Source: CAD feature listing. Evaluate the final solid. Frame: model axes, mm. A direction names the side the tool comes from. Coordinates: 2 decimals unless noted, no trailing zeros. Loops run counter-clockwise (first coordinate to the right, second up) from the corner with the lowest first, then second, coordinate; pieces in that order, holes last. Notation, with made-up numbers: (-2, -7) -> (4, -7) arc R10 cw to (4, 4) -> close; hole circle Ø6 at (67, 42.25). An arc over 180 degrees is marked (long way). Answer as a JSON object with one key per item and string values. Group by question number.
from build123d import *


with BuildPart() as part:
    # Sketch1 → Revolve1 (revolve)
    with BuildSketch(Plane.XY, mode=Mode.PRIVATE) as revolve1_sk:
        with BuildLine():
            Line((0, 76.2), (-7.9375, 76.2))
            Line((-7.9375, 76.2), (-7.9375, 64.29375))
            ThreePointArc((-7.9375, 64.29375), (-8.169983992, 63.732483992), (-8.73125, 63.5))
            Line((-8.73125, 63.5), (-12.7, 63.5))
            Line((-12.7, 63.5), (-12.7, -63.5))
            Line((-12.7, -63.5), (-8.73125, -63.5))
            ThreePointArc((-8.73125, -63.5), (-8.169983992, -63.732483992), (-7.9375, -64.29375))
            Line((-7.9375, -64.29375), (-7.9375, -76.2))
            Line((-7.9375, -76.2), (0, -76.2))
            Line((0, -76.2), (0, 76.2))
        make_face()
    revolve(revolve1_sk.sketch.rotate(Axis((0, 76.2, 0), (0, -1, 0)), 270), axis=Axis((0, 76.2, 0), (0, -1, 0)))


solid = part.part
1. Section query B-B on x = 0. Return loops of the section in (y, z), then the cut area to 3 significant figures.
2. Reachability of faces 1 (the face through (7.7, -0.9, -10.1)), 2 (the face through (-9, -63.5, 3)), 3 (the face through (-9, 63.5, -3)) from +Z, -Z, +X, -X, +Y, -Y: full face, straight path, thin tool, end or side. Return the list, or none.
3. Section query A-A on z = 0. Return loops of the section in (x, y), then the cut area to 3 significant figures.
4. Ray query, L1, parallel to Y at x = -1.25, z = 8.5; L2, parallel to Z at x = -10.75, y = -28.5; L3, parallel to Z at x = -10.5, y = 37. Return the intervals inside material, ascending.
5. Section query C-C on y = 17. Return loops of the section in (x, z), then the cut area to 3 significant figures.
6. Pin query (flat end, axial travel): pin 1 Ø2 at (y, z) = (-1, -1.5) entering from -X; pin 2 Ø3 at (y, z) = (-22, -8) entering from +X; pin 3 Ø8 at (y, z) = (-46, 7) entering from +X. Return the tip coordinate at first contact, or that it passes through.
Solved:
{
 "1": {"outline": "(-76.2, -7.94) -> (-64.29, -7.94) arc R0.79 cw to (-63.5, -8.73) -> (-63.5, -12.7) -> (63.5, -12.7) -> (63.5, -8.73) arc R0.79 cw to (64.29, -7.94) -> (76.2, -7.94) -> (76.2, 7.94) -> (64.29, 7.94) arc R0.79 cw to (63.5, 8.73) -> (63.5, 12.7) -> (-63.5, 12.7) -> (-63.5, 8.73) arc R0.79 cw to (-64.29, 7.94) -> (-76.2, 7.94) -> close", "area": "3,630 mm^2"},
 "2": {"face 1": "+Y, -Y", "face 2": "-Y", "face 3": "+Y"},
 "3": {"outline": "(-12.7, -63.5) -> (-8.73, -63.5) arc R0.79 cw to (-7.94, -64.29) -> (-7.94, -76.2) -> (7.94, -76.2) -> (7.94, -64.29) arc R0.79 cw to (8.73, -63.5) -> (12.7, -63.5) -> (12.7, 63.5) -> (8.73, 63.5) arc R0.79 cw to (7.94, 64.29) -> (7.94, 76.2) -> (-7.94, 76.2) -> (-7.94, 64.29) arc R0.79 cw to (-8.73, 63.5) -> (-12.7, 63.5) -> close", "area": "3,630 mm^2"},
 "4": {"L1": "-63.51 to 63.51", "L2": "-6.76 to 6.76", "L3": "-7.14 to 7.14"},
 "5": {"outline": "circle Ø25.4 at (0, 0)", "area": "507 mm^2"},
 "6": {"pin 1": "x = -12.69", "pin 2": "x = 10.91", "pin 3": "x = 12.34"}
}
